Geometry: final body of the model. Coordinates: model frame, mm. A direction names the side the tool comes from. Give positions to 0.01 mm unless a question says otherwise; leave off trailing zeros. Loops run counter-clockwise (first coordinate to the right, second up) from the corner with the lowest first, then second, coordinate; pieces in that order, holes last.
1. Section A-A, the plane x = 35. Output: boundary loops of the cut face in (y, z), then the cut area to 4 significant figures.
2. Material intervals for line 1 along Y through (x, z) = (17.5, 15.25); line 2 along Z through (x, y) = (-6, 9), sorted ascending.
3. Section D-D, the plane z = 14.75. Output: boundary loops of the cut face in (x, y).
4. Access query for faces 1 (the face through (-1, -31.5, 9)), 2 (the face through (-1, -39, 16)). Directions: +Z, -Z, +X, -X, +Y, -Y. A direction counts if a zero-diameter tool reaches every point of the face in a straight line with its end or side. Return the directions, or none.
5. Section B-B, the plane x = -7. Output: boundary loops of the cut face in (y, z), then the cut area to 3 significant figures.
6. Draft query along Y for faces 3 (the face through (35.98, 34.71, 1.01)), 4 (the face through (-1, 1, 0)), 5 (the face through (-1, 47.5, 1)). Return one class per face: +Y half, -Y half, draft (parallel to the pull), parting line (faces both ways), or undercut.
7. First-contact query: P1, Ø3, axis at x = -34.975, y = 33.125, coming from the -Z side; P2, Ø4, axis at x = -4, z = 6.5, coming from the +Y side. Flat tips, straight axial feed; report the tip coordinate or a pass-through.
8. Section C-C, the plane y = -27. Output: boundary loops of the cut face in (x, z), then the cut area to 3 significant figures.
from build123d import *

# Parameters (mm, degrees)
F0_W     = 89.7
F0_H     = 95
F1_DEPTH = 2
F2_R     = 1.875
F3_DEPTH = 2.001
F4_W     = 89.7
F4_H     = 16
F5_DEPTH = 14


with BuildPart() as f1:
    # F0 (on Top) → F1 (new body)
    with BuildSketch(Plane.XY):
        Rectangle(F0_W, F0_H)
    extrude(amount=F1_DEPTH)

    # F2 (on face) → F3 (cut, through all)
    with BuildSketch(Plane.XY.offset(2)):
        with Locations((-34.975, 33.125)):
            Circle(F2_R)
        with Locations((34.975, 33.125)):
            Circle(F2_R)
    extrude(amount=-F3_DEPTH, mode=Mode.SUBTRACT)

    # F4 (on face) → F5 (join)
    with BuildSketch(Plane.XY.offset(2)):
        with Locations((0, -39.5)):
            Rectangle(F4_W, F4_H)
    extrude(amount=F5_DEPTH)


solid = f1.part
Answers below:
1. outline: (-47.5, 0) - (31.25, 0) - (31.25, 2) - (-31.5, 2) - (-31.5, 16) - (-47.5, 16) - close; (35, 0) - (47.5, 0) - (47.5, 2) - (35, 2) - close
1. area: 406.5 mm2
2. line 1: y = -47.5 to -31.5
2. line 2: z = 0 to 2
3. outline: (-44.85, -47.5) - (44.85, -47.5) - (44.85, -31.5) - (-44.85, -31.5) - close
4. face 1: +Z, +X, -X, +Y
4. face 2: +Z, +X, -X, +Y, -Y
5. outline: (-47.5, 0) - (47.5, 0) - (47.5, 2) - (-31.5, 2) - (-31.5, 16) - (-47.5, 16) - close
5. area: 414 mm2
6. face 3: undercut
6. face 4: draft
6. face 5: +Y half
7. P1: passes through
7. P2: stops at y = -31.5
8. outline: (-44.85, 0) - (44.85, 0) - (44.85, 2) - (-44.85, 2) - close
8. area: 179 mm2
